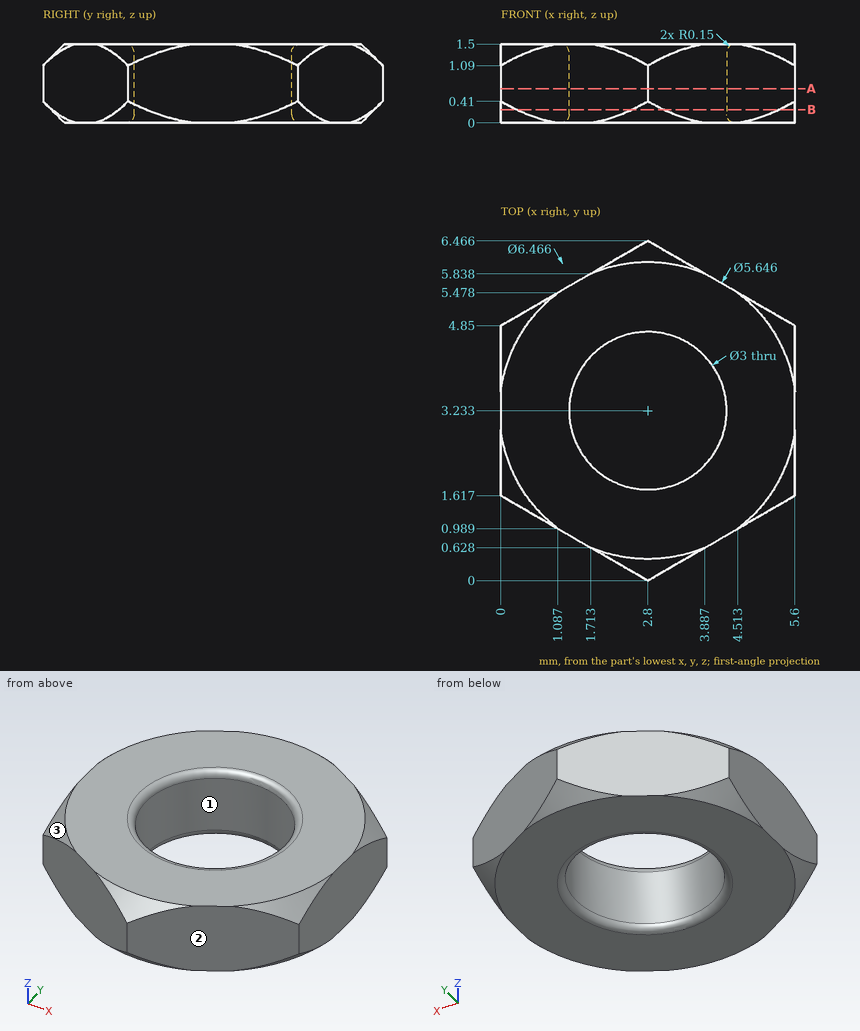
Geometry check sheet. Reference: drawing and pictorial views, mm from the part's lowest x, y, z. Round coordinates to 2 decimals unless told otherwise and drop trailing zeros. Order: outer loops, then holes, each group sorted by start corner. A loop starts at its lowest first (then second) coordinate and runs counter-clockwise, first axis right, second up. Notation, with made-up numbers: (69, 21.5) - (89, 21.5) arc R9 ccw to (89, 28.5) - close; hole circle Ø2 at (-2.5, 78). An arc over 180 degrees is marked (long way). One line per question, with ' | ' between items. Start each with the question number.
(1) Sectioned sample at B-B on z = 0.25. Record the cut outline in (x, y) (1 decimal), and give its area (3 significant figures).
(2) Thickness scan on L1, parallel to X at y = 3.25, z = 0.8; L2, parallel to Y at x = 2.05, z = 0.1 (1 decimal); L3, parallel to Y at x = 3.3, z = 1.3. Record the ranges inside material, lowest first. Write a range as [from, to].
(3) Release check for a two-part mould opening along X. For the marked faces 1, 2 and 3 record: released by +X, released by -X, zero draft, split by the parting line, or undercut.
(4) Depth check by flat-ended pin: pin 1 Ø1.8 at (x, y) = (2.8, 3.23) entering from +Z. Enter the tip coordinate at first touch or a pass-through.
(5) Sectioned sample at A-A on z = 0.65. Record the cut outline in (x, y).
Conclusion:
1) outline: (0, 2) arc R3.1 ccw to (0.3, 1.4) - (2.5, 0.2) arc R3.1 ccw to (3.1, 0.2) - (5.3, 1.4) arc R3.1 ccw to (5.6, 2) - (5.6, 4.5) arc R3.1 ccw to (5.3, 5) - (3.1, 6.3) arc R3.1 ccw to (2.5, 6.3) - (0.3, 5) arc R3.1 ccw to (0, 4.5) - close; hole circle Ø3 at (2.8, 3.2) | area: 19.8 mm2
2) L1: x = [0, 1.3], [4.3, 5.6] | L2: y = [0.4, 1.9], [4.5, 6] | L3: y = [0.29, 1.82], [4.65, 6.18]
3) face 1: undercut | face 2: released by +X | face 3: released by -X
4) pin 1: passes through
5) outline: (0, 1.62) - (2.8, 0) - (5.6, 1.62) - (5.6, 4.85) - (2.8, 6.47) - (0, 4.85) - close; hole circle Ø3 at (2.8, 3.23)
